Can you work these out from the model? Positions are in its coordinate system, mm. Face numbers are marked on the shaded views. Coordinates: 2 decimals unless noted, no trailing zeros. Loops run counter-clockwise (first coordinate to the right, second up) from the corner with the lowest first, then second, coordinate; pieces in that order, holes last. Notation, with made-up numbers: (18.25, 13) - (32.25, 13) arc R19 cw to (32.25, 28) - close; hole circle Ø3 at (74, 5). An arc over 180 degrees is marked (long way). Put each result on its own line as item: value. Start each with the question number.
from build123d import *

# Parameters (mm, degrees)
F0_R         = 5
F1_DEPTH     = 3
F2_C1_SIZE2  = 0.75
F2_C1_SIZE   = 2
F2_C2_SIZE2  = 0.75
F2_C2_SIZE   = 2
F2_C3_SIZE2  = 0.75
F2_C3_SIZE   = 2
F2_C4_SIZE2  = 0.75
F2_C4_SIZE   = 2
F2_C5_SIZE2  = 0.75
F2_C5_SIZE   = 2
F2_C6_SIZE2  = 0.75
F2_C6_SIZE   = 2
F2_C7_SIZE2  = 0.75
F2_C7_SIZE   = 2
F2_C8_SIZE2  = 0.75
F2_C8_SIZE   = 2
F2_C9_SIZE2  = 2
F2_C9_SIZE   = 0.75
F2_C10_SIZE2 = 0.75
F2_C10_SIZE  = 2
F2_C11_SIZE2 = 0.75
F2_C11_SIZE  = 2
F2_C12_SIZE2 = 0.75
F2_C12_SIZE  = 2
F2_C13_SIZE2 = 0.75
F2_C13_SIZE  = 2
F2_C14_SIZE2 = 0.75
F2_C14_SIZE  = 2
F2_C15_SIZE2 = 0.75
F2_C15_SIZE  = 2
F2_C16_SIZE2 = 0.75
F2_C16_SIZE  = 2
F4_SIZE      = 0.5


# Not quite as in the source:
# - two fillets or chamfers of one size are made in one step


with BuildPart() as f1:
    # F0 (on Front) → F1 (new body)
    with BuildSketch(Plane.XZ):
        with BuildLine():
            ThreePointArc((14.98661002, -0.6336561441), (10.7222272749, 2.4563880526), (13.2160968729, 7.0947010823))
            ThreePointArc((13.2160968729, 7.0947010823), (12.2264008787, 8.6899437025), (11.0451961285, 10.1490710157))
            ThreePointArc((11.0451961285, 10.1490710157), (5.8448309663, 9.3186882647), (4.3284804738, 14.3619029654))
            ThreePointArc((4.3284804738, 14.3619029654), (2.5006528507, 14.790089091), (0.6336561441, 14.98661002))
            ThreePointArc((0.6336561441, 14.98661002), (0.6461967949, 14.8041057756), (0.6503799283, 14.6212190113))
            ThreePointArc((0.6503799283, 14.6212190113), (-2.6355906754, 10.6854646971), (-7.0947010823, 13.2160968729))
            ThreePointArc((-7.0947010823, 13.2160968729), (-8.6899437025, 12.2264008787), (-10.1490710157, 11.0451961285))
            ThreePointArc((-10.1490710157, 11.0451961285), (-9.0856364951, 9.6683222969), (-8.7073021792, 7.970224045))
            ThreePointArc((-8.7073021792, 7.970224045), (-10.5414770644, 4.6073084094), (-14.3619029654, 4.3284804738))
            ThreePointArc((-14.3619029654, 4.3284804738), (-14.790089091, 2.5006528507), (-14.98661002, 0.6336561441))
            ThreePointArc((-14.98661002, 0.6336561441), (-11.9250702797, -0.3948303977), (-10.6212190113, -3.3496200717))
            ThreePointArc((-10.6212190113, -3.3496200717), (-11.3333254186, -5.6277236082), (-13.2160968729, -7.0947010823))
            ThreePointArc((-13.2160968729, -7.0947010823), (-12.2264008787, -8.6899437025), (-11.0451961285, -10.1490710157))
            ThreePointArc((-11.0451961285, -10.1490710157), (-6.6100564697, -8.9456610257), (-3.970224045, -12.7073021792))
            ThreePointArc((-3.970224045, -12.7073021792), (-4.060813969, -13.5537730042), (-4.3284804738, -14.3619029654))
            ThreePointArc((-4.3284804738, -14.3619029654), (-2.5006528507, -14.790089091), (-0.6336561441, -14.98661002))
            ThreePointArc((-0.6336561441, -14.98661002), (2.4563880526, -10.7222272749), (7.0947010823, -13.2160968729))
            ThreePointArc((7.0947010823, -13.2160968729), (8.6899437025, -12.2264008787), (10.1490710157, -11.0451961285))
            ThreePointArc((10.1490710157, -11.0451961285), (9.3186882647, -5.8448309663), (14.3619029654, -4.3284804738))
            ThreePointArc((14.3619029654, -4.3284804738), (14.790089091, -2.5006528507), (14.98661002, -0.6336561441))
        make_face()
        Circle(F0_R, mode=Mode.SUBTRACT)
    extrude(amount=F1_DEPTH)

    # F2: chamfer of 2 x 0.75 on 16 edges, made by hand

    # F2_c1
    f2_c1_edges = [f1.edges().sort_by_distance(p)[0] for p in [
        (8.6899437025, -3, -12.2264008787),
    ]]
    f2_c1_side = f1.faces().sort_by_distance((8.6812537588, -3, -12.2141744779))[0]
    chamfer(f2_c1_edges, length=F2_C1_SIZE, length2=F2_C1_SIZE2, reference=f2_c1_side)

    # F2_c2
    f2_c2_edges = [f1.edges().sort_by_distance(p)[0] for p in [
        (14.790089091, -3, -2.5006528507),
    ]]
    f2_c2_side = f1.faces().sort_by_distance((14.7752990019, -3, -2.4981521978))[0]
    chamfer(f2_c2_edges, length=F2_C2_SIZE, length2=F2_C2_SIZE2, reference=f2_c2_side)

    # F2_c3
    f2_c3_edges = [f1.edges().sort_by_distance(p)[0] for p in [
        (12.2264008787, -3, 8.6899437025),
    ]]
    f2_c3_side = f1.faces().sort_by_distance((12.2141744779, -3, 8.6812537588))[0]
    chamfer(f2_c3_edges, length=F2_C3_SIZE, length2=F2_C3_SIZE2, reference=f2_c3_side)

    # F2_c4
    f2_c4_edges = [f1.edges().sort_by_distance(p)[0] for p in [
        (2.5006528507, -3, 14.790089091),
    ]]
    f2_c4_side = f1.faces().sort_by_distance((2.4981521978, -3, 14.7752990019))[0]
    chamfer(f2_c4_edges, length=F2_C4_SIZE, length2=F2_C4_SIZE2, reference=f2_c4_side)

    # F2_c5
    f2_c5_edges = [f1.edges().sort_by_distance(p)[0] for p in [
        (-8.6899437025, -3, 12.2264008787),
    ]]
    f2_c5_side = f1.faces().sort_by_distance((-8.6812537588, -3, 12.2141744779))[0]
    chamfer(f2_c5_edges, length=F2_C5_SIZE, length2=F2_C5_SIZE2, reference=f2_c5_side)

    # F2_c6
    f2_c6_edges = [f1.edges().sort_by_distance(p)[0] for p in [
        (-14.790089091, -3, 2.5006528507),
    ]]
    f2_c6_side = f1.faces().sort_by_distance((-14.7752990019, -3, 2.4981521978))[0]
    chamfer(f2_c6_edges, length=F2_C6_SIZE, length2=F2_C6_SIZE2, reference=f2_c6_side)

    # F2_c7
    f2_c7_edges = [f1.edges().sort_by_distance(p)[0] for p in [
        (-12.2264008787, -3, -8.6899437025),
    ]]
    f2_c7_side = f1.faces().sort_by_distance((-12.2141744779, -3, -8.6812537588))[0]
    chamfer(f2_c7_edges, length=F2_C7_SIZE, length2=F2_C7_SIZE2, reference=f2_c7_side)

    # F2_c8
    f2_c8_edges = [f1.edges().sort_by_distance(p)[0] for p in [
        (-2.5006528507, -3, -14.790089091),
    ]]
    f2_c8_side = f1.faces().sort_by_distance((-2.4981521978, -3, -14.7752990019))[0]
    chamfer(f2_c8_edges, length=F2_C8_SIZE, length2=F2_C8_SIZE2, reference=f2_c8_side)

    # F2_c9
    f2_c9_edges = [f1.edges().sort_by_distance(p)[0] for p in [
        (-12.2264008787, 0, -8.6899437025),
    ]]
    f2_c9_side = f1.faces().sort_by_distance((-12.2264008787, -0.015, -8.6899437025))[0]
    chamfer(f2_c9_edges, length=F2_C9_SIZE, length2=F2_C9_SIZE2, reference=f2_c9_side)

    # F2_c10
    f2_c10_edges = [f1.edges().sort_by_distance(p)[0] for p in [
        (-14.790089091, 0, 2.5006528507),
    ]]
    f2_c10_side = f1.faces().sort_by_distance((-14.7752990019, 0, 2.4981521978))[0]
    chamfer(f2_c10_edges, length=F2_C10_SIZE, length2=F2_C10_SIZE2, reference=f2_c10_side)

    # F2_c11
    f2_c11_edges = [f1.edges().sort_by_distance(p)[0] for p in [
        (-8.6899437025, 0, 12.2264008787),
    ]]
    f2_c11_side = f1.faces().sort_by_distance((-8.6812537588, 0, 12.2141744779))[0]
    chamfer(f2_c11_edges, length=F2_C11_SIZE, length2=F2_C11_SIZE2, reference=f2_c11_side)

    # F2_c12
    f2_c12_edges = [f1.edges().sort_by_distance(p)[0] for p in [
        (2.5006528507, 0, 14.790089091),
    ]]
    f2_c12_side = f1.faces().sort_by_distance((2.4981521978, 0, 14.7752990019))[0]
    chamfer(f2_c12_edges, length=F2_C12_SIZE, length2=F2_C12_SIZE2, reference=f2_c12_side)

    # F2_c13
    f2_c13_edges = [f1.edges().sort_by_distance(p)[0] for p in [
        (12.2264008787, 0, 8.6899437025),
    ]]
    f2_c13_side = f1.faces().sort_by_distance((12.2141744779, 0, 8.6812537588))[0]
    chamfer(f2_c13_edges, length=F2_C13_SIZE, length2=F2_C13_SIZE2, reference=f2_c13_side)

    # F2_c14
    f2_c14_edges = [f1.edges().sort_by_distance(p)[0] for p in [
        (14.790089091, 0, -2.5006528507),
    ]]
    f2_c14_side = f1.faces().sort_by_distance((14.7752990019, 0, -2.4981521978))[0]
    chamfer(f2_c14_edges, length=F2_C14_SIZE, length2=F2_C14_SIZE2, reference=f2_c14_side)

    # F2_c15
    f2_c15_edges = [f1.edges().sort_by_distance(p)[0] for p in [
        (8.6899437025, 0, -12.2264008787),
    ]]
    f2_c15_side = f1.faces().sort_by_distance((8.6812537588, 0, -12.2141744779))[0]
    chamfer(f2_c15_edges, length=F2_C15_SIZE, length2=F2_C15_SIZE2, reference=f2_c15_side)

    # F2_c16
    f2_c16_edges = [f1.edges().sort_by_distance(p)[0] for p in [
        (-2.5006528507, 0, -14.790089091),
    ]]
    f2_c16_side = f1.faces().sort_by_distance((-2.4981521978, 0, -14.7752990019))[0]
    chamfer(f2_c16_edges, length=F2_C16_SIZE, length2=F2_C16_SIZE2, reference=f2_c16_side)

    # F4
    f4_edges = [f1.edges().sort_by_distance(p)[0] for p in [
        (-5, -3, 0),
        (-5, 0, 0),
    ]]
    chamfer(f4_edges, length=F4_SIZE)


solid = f1.part
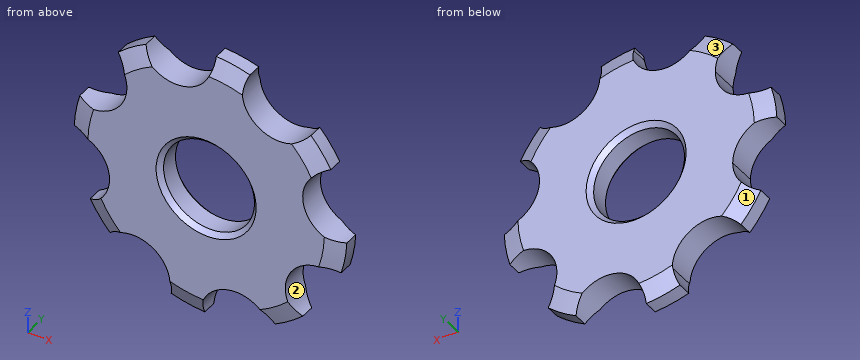
Q1. I want a section at A-A on y = -1.2. List the corners of the cut face in (x, z) for me, and give its area (3 significant figures).
Q2. We'd pull the mould along Z, two halves only. Please class the marked faces 1, 2 and 3: released by +Z, released by -Z, zero draft, split by the parting line, or undercut.
Q3. Will these pins go through, and if not, where does the flat tip stop? pin 1 (1.5 mm diameter, centred on x = -2, y = -1.5, fed in from +Z); pin 2 (9 mm diameter, centred on x = 0, z = 0, fed in from +Y).
Q4. Please list where these lines run through material, in increasing order: line 1 along Z through (x, y) = (0, -1.9); line 2 along X through (y, z) = (-0.05, 0.25); line 3 along X through (y, z) = (-1.45, -9.5). Write a range as [from, to].
Calculated:
1. outline: (-14.99, 0.63) arc R4 cw to (-13.22, -7.09) arc R15 ccw to (-11.05, -10.15) arc R4 cw to (-4.33, -14.36) arc R15 ccw to (-0.63, -14.99) arc R4 cw to (7.09, -13.22) arc R15 ccw to (10.15, -11.05) arc R4 cw to (14.36, -4.33) arc R15 ccw to (14.99, -0.63) arc R4 cw to (13.22, 7.09) arc R15 ccw to (11.05, 10.15) arc R4 cw to (4.33, 14.36) arc R15 ccw to (0.63, 14.99) arc R4 cw to (-7.09, 13.22) arc R15 ccw to (-10.15, 11.05) arc R4 cw to (-14.36, 4.33) arc R15 ccw to start; hole circle Ø10 at (0, 0)
1. area: 439 mm2
2. face 1: released by -Z
2. face 2: undercut
2. face 3: released by +Z
3. pin 1: z = 11.22
3. pin 2: through
4. line 1: [-12.43, -5], [5, 12.43]
4. line 2: [-12.88, -5.44], [5.44, 12.09]
4. line 3: [-11.61, -10.36], [-5.58, 9.01]
